Job drawing, mm, ordinate dimensions from the low corner. One solid piece. A direction names the side the tool comes from. Give positions to 0.01 mm unless a question says otherwise; leave off trailing zeros. Order: outer loops, then holes, each group sorted by start corner. A loop starts at its lowest first (then second) coordinate and runs counter-clockwise, first axis right, second up. Notation, with made-up numbers: M 61,-11.5 L 98,-11.5 A24 ccw 98,-0.5 Z; hole C 57,-27.5 d4. An arc over 180 degrees is marked long. Put each result on its own line as item: value. Start each with the question number.
1) Pin check, flat tips, straight feed: pin 1 (6 mm diameter, centred on x = 45.5, y = 38, fed in from +Z); pin 2 (2 mm diameter, centred on x = 18.5, z = 1.5, fed in from -Y); pin 3 (4.5 mm diameter, centred on x = 66, z = 9.5, fed in from +Y). Stop position of each tip, or through.
2) Drill centre lines: line 1 (X direction, y = 10, z = 1.5); line 2 (Y direction, x = 4, z = 8.25). Where is each one in solid material? Low to high. Write a range as [from, to].
3) Cut at C-C (x = 62.5). Write the cut outline in (y, z), and give its area (3 significant figures).
4) Cut at D-D (y = 30.5). Write the cut outline in (x, z).
5) Tool access for the marked faces 1 and 2: list every direction of +Z, -Z, +X, -X, +Y, -Y with a clear straight run to the whole face (end or side of a thin tool).
6) Cut at B-B (z = 5.5). Write the cut outline in (x, y), and give its area (3 significant figures).
7) Cut at A-A (y = 24). Write the cut outline in (x, z), and give its area (3 significant figures).
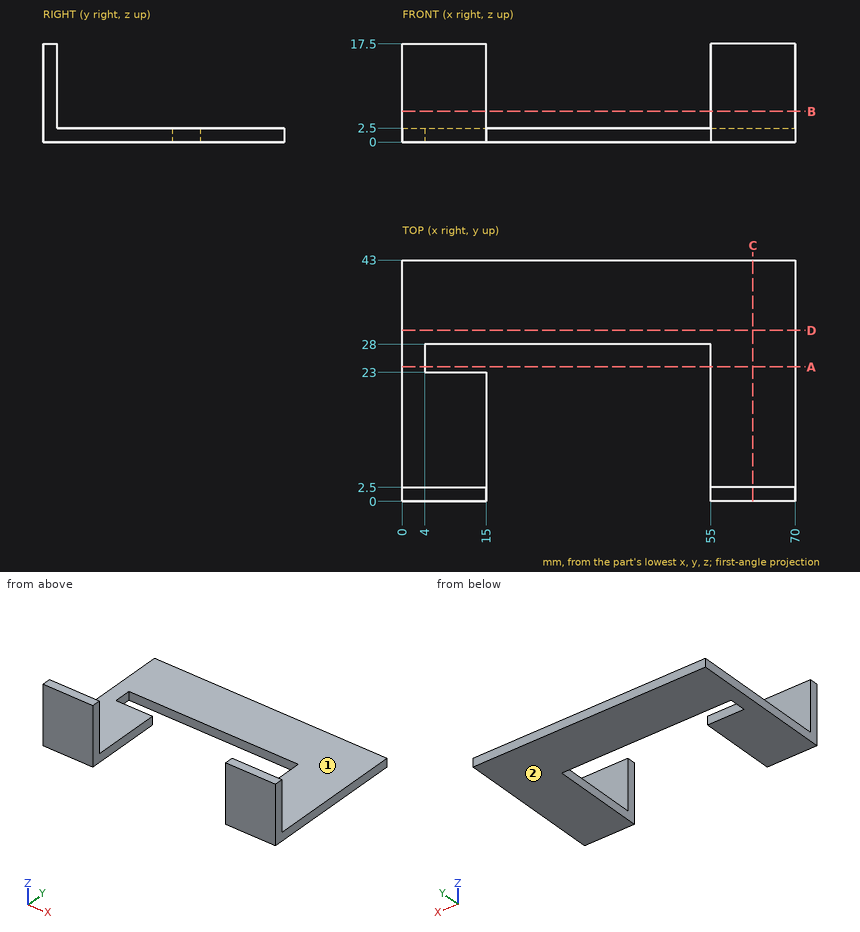
Solution:
1. pin 1: z = 2.5
1. pin 2: y = 28
1. pin 3: y = 2.5
2. line 1: [0, 15], [55, 70]
2. line 2: [0, 2.5]
3. outline: M 0,0 L 43,0 L 43,2.5 L 2.5,2.5 L 2.5,17.5 L 0,17.5 Z
3. area: 145 mm²
4. outline: M 0,0 L 70,0 L 70,2.5 L 0,2.5 Z
5. face 1: +Z, +X, -X, +Y
5. face 2: -Z, +X, -X, +Y, -Y
6. outline: M 0,0 L 15,0 L 15,2.5 L 0,2.5 Z; M 55,0 L 70,0 L 70,2.5 L 55,2.5 Z
6. area: 75.0 mm²
7. outline: M 0,0 L 4,0 L 4,2.5 L 0,2.5 Z; M 55,0 L 70,0 L 70,2.5 L 55,2.5 Z
7. area: 47.5 mm²
